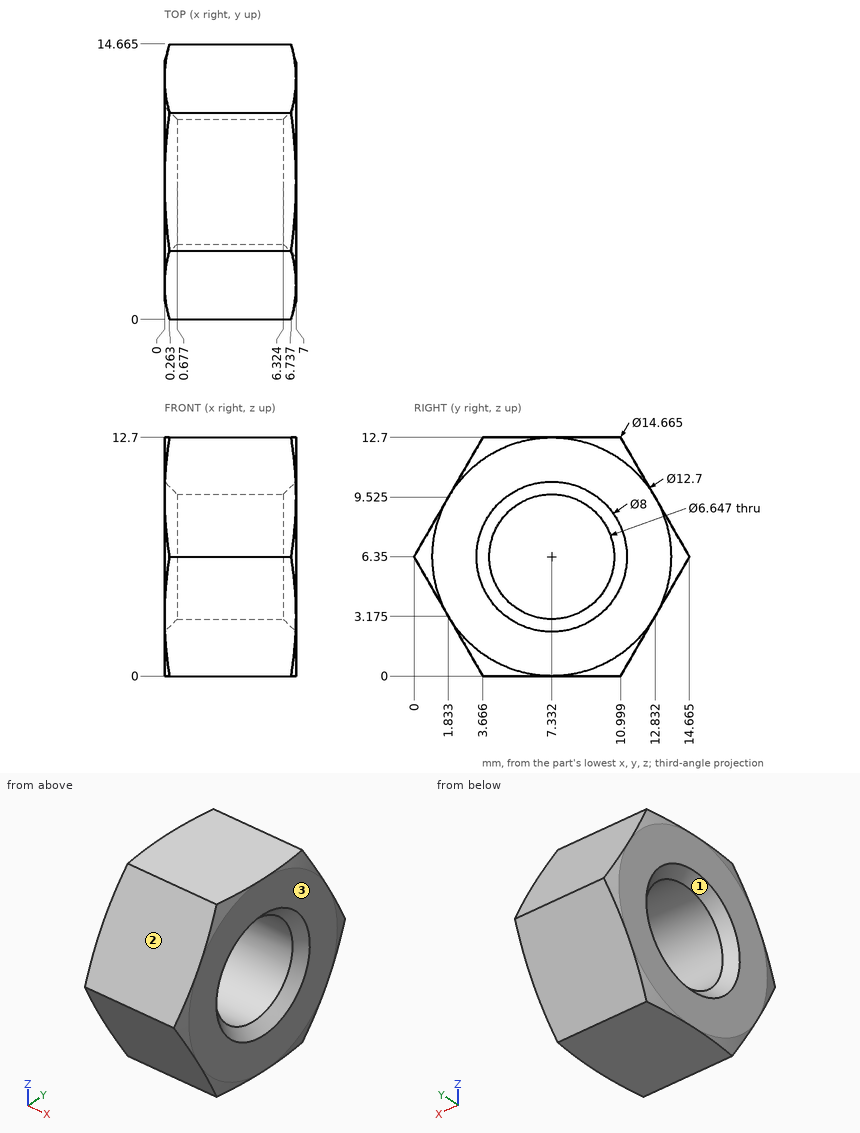
The drawing under review shows one solid part. Ordinate dimensions are in mm from its lowest x, y, z. Coordinates: 2 decimals unless noted, no trailing zeros. Answer as a JSON object with one key per item and string values.
Q1. Clearance check with flat-ended pins moving along their axes: pin 1 Ø1.5 at (x, z) = (2.5, 8) entering from +Y (1 decimal); pin 2 Ø5.5 at (y, z) = (7.33, 6.35) entering from -X. State where each tip first meets the part, or that it passes through.
Answer block:
{"pin 1": "stops at y = 14.1", "pin 2": "passes through"}
Q2. To check wall thickness, follow L1, parallel to Y at x = 1.75, z = 4.75 (1 decimal); L2, parallel to Z at x = 5.5, y = 4.5 (1 decimal); L3, parallel to Z at x = 5.75, y = 5.5 (1 decimal). State the ranges of each line that lie inside material, in increasing order.
Answer block:
{"L1": "y = 0.9 to 4.4, 10.2 to 13.7", "L2": "z = 0 to 4.6, 8.1 to 12.7", "L3": "z = 0 to 3.6, 9.1 to 12.7"}
Q3. The part is to be moulded in two halves that separate along Y. For the marked faces 1, 2 and 3, say which applies: +Y half, -Y half, draft (parallel to the pull), parting line (faces both ways), or undercut.
Answer block:
{"face 1": "undercut", "face 2": "-Y half", "face 3": "draft"}
